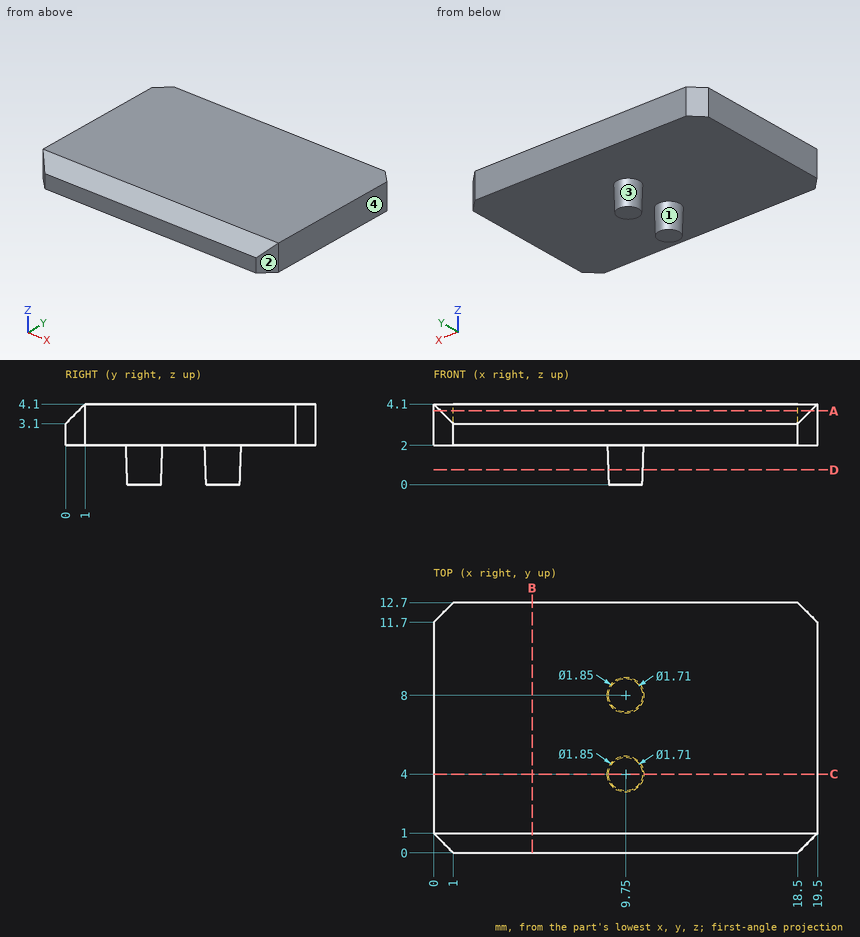
Geometry check sheet. Reference: drawing and pictorial views, mm from the part's lowest x, y, z. Round coordinates to 2 decimals unless told otherwise and drop trailing zeros. Order: outer loops, then holes, each group sorted by start corner. A loop starts at its lowest first (then second) coordinate and runs counter-clockwise, first axis right, second up. Notation, with made-up numbers: (50.5, 74.25) - (58.5, 74.25) arc R28 ccw to (58.5, 102.25) - close; hole circle Ø2 at (16, 85.5). An arc over 180 degrees is marked (long way). One line per question, with ' | ' between items. Start each with the question number.
(1) Release check for a two-part mould opening along Y. For the marked faces 1, 2, 3 and 4 record: released by +Y, released by -Y, zero draft, split by the parting line, or undercut.
(2) Sectioned sample at C-C on y = 4. Record the cut outline in (x, z) (1 decimal), and give its area (3 significant figures).
(3) Sectioned sample at A-A on z = 3.75. Record the cut outline in (x, y), and give its area (3 significant figures).
(4) Thickness scan on L1, parallel to Z at x = 15.75, y = 2.25; L2, parallel to Y at x = 9.75, z = 0.3 (1 decimal); L3, parallel to Y at x = 10.25, z = 0.2. Record the ranges inside material, lowest first. Write a range as [from, to].
(5) Sectioned sample at D-D on z = 0.75. Record the cut outline in (x, y).
(6) Sectioned sample at B-B on x = 5. Record the cut outline in (y, z).
(7) Depth check by flat-ended pin: pin 1 Ø4 at (x, y) = (5.5, 4) entering from -Z. Enter the tip coordinate at first touch or a pass-through.
Conclusion:
1) face 1: undercut | face 2: released by -Y | face 3: undercut | face 4: zero draft
2) outline: (0, 2) - (8.8, 2) - (8.9, 0) - (10.6, 0) - (10.7, 2) - (19.5, 2) - (19.5, 4.1) - (0, 4.1) - close | area: 44.5 mm2
3) outline: (0, 1) - (0.35, 0.65) - (19.15, 0.65) - (19.5, 1) - (19.5, 11.7) - (18.5, 12.7) - (1, 12.7) - (0, 11.7) - close | area: 234 mm2
4) L1: z = [2, 4.1] | L2: y = [3.1, 4.9], [7.1, 8.9] | L3: y = [3.3, 4.7], [7.3, 8.7]
5) outline: circle Ø1.76 at (9.75, 4); circle Ø1.76 at (9.75, 8)
6) outline: (0, 2) - (12.7, 2) - (12.7, 4.1) - (1, 4.1) - (0, 3.1) - close
7) pin 1: stops at z = 2
